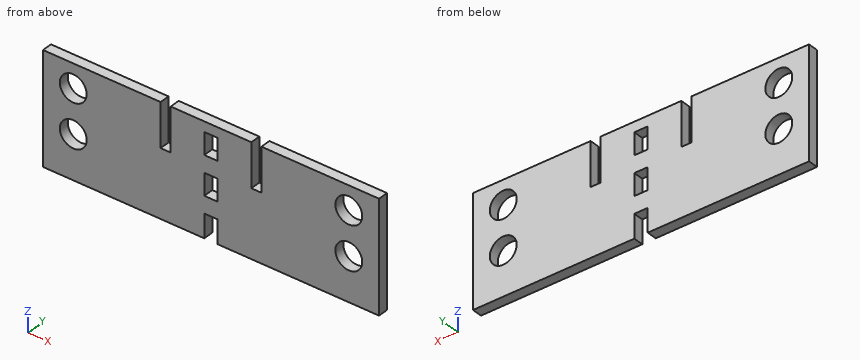
```python
from build123d import *

# Parameters (mm, degrees)
SKETCH_1_R          = 4
EXTRUDE_1_DEPTH     = 3
SKETCH_2_W          = 4
SKETCH_2_H          = 3
CUT_EXTRUDE_1_DEPTH = 3.33
SKETCH_3_W          = 24
SKETCH_3_H          = 13
EXTRUDE_2_DEPTH     = 3
SKETCH_4_W          = 35
SKETCH_4_H          = 13
EXTRUDE_3_DEPTH     = 3
SKETCH_5_R          = 4
CUT_EXTRUDE_2_DEPTH = 25
SKETCH_6_W          = 4
SKETCH_6_H          = 6.5
CUT_EXTRUDE_3_DEPTH = 25


with BuildPart() as part:
    # Эскиз1 → Бобышка-Вытянуть1 (new body)
    with BuildSketch(Plane(origin=(0, 0, 0), x_dir=(1, 0, 0), z_dir=(0, 1, 0))):
        Polygon((2, 10), (50, 10), (50, -10), (-50, -10), (-50, 10), (-2, 10), (-2, 6.32739691), (2, 6.32739691), align=None)
        with Locations(Location((-41, -3, 0), (0, 0, 270))):
            Circle(SKETCH_1_R, mode=Mode.SUBTRACT)
        with Locations(Location((41, -3, 0), (0, 0, 90))):
            Circle(SKETCH_1_R, mode=Mode.SUBTRACT)
    extrude(amount=EXTRUDE_1_DEPTH)

    # Эскиз2 → Вырез-Вытянуть1 (cut)
    with BuildSketch(Plane(origin=(0, 0, -6.32739691), x_dir=(-1, 0, 0), z_dir=(0, 0, -1))):
        with Locations((0, 1.5)):
            Rectangle(SKETCH_2_W, SKETCH_2_H)
    extrude(amount=-CUT_EXTRUDE_1_DEPTH, mode=Mode.SUBTRACT)

    # Эскиз3 → Бобышка-Вытянуть2 (add)
    with BuildSketch(Plane(origin=(0, 3, 0), x_dir=(1, 0, 0), z_dir=(0, 1, 0))):
        with Locations((0, -16.5)):
            Rectangle(SKETCH_3_W, SKETCH_3_H)
    extrude(amount=-EXTRUDE_2_DEPTH)

    # Эскиз4 → Бобышка-Вытянуть3 (add)
    with BuildSketch(Plane(origin=(0, 3, 0), x_dir=(1, 0, 0), z_dir=(0, 1, 0))):
        with Locations((-32.5, -16.5)):
            Rectangle(SKETCH_4_W, SKETCH_4_H)
        with Locations((32.5, -16.5)):
            Rectangle(SKETCH_4_W, SKETCH_4_H)
    extrude(amount=-EXTRUDE_3_DEPTH)

    # Эскиз5 → Вырез-Вытянуть2 (cut)
    with BuildSketch(Plane(origin=(0, 3, 0), x_dir=(1, 0, 0), z_dir=(0, 1, 0))):
        with Locations(Location((-41, -15.92753052, 0), (0, 0, 270))):
            Circle(SKETCH_5_R)
        with Locations(Location((41, -15.92753052, 0), (0, 0, 270))):
            Circle(SKETCH_5_R)
    extrude(amount=-CUT_EXTRUDE_2_DEPTH, mode=Mode.SUBTRACT)

    # Эскиз6 → Вырез-Вытянуть3 (cut)
    with BuildSketch(Plane(origin=(0, 3, 0), x_dir=(1, 0, 0), z_dir=(0, 1, 0))):
        with Locations((0, -5.25260309)):
            Rectangle(SKETCH_6_W, SKETCH_6_H)
        with Locations((0, -16.75260309)):
            Rectangle(SKETCH_6_W, SKETCH_6_H)
    extrude(amount=-CUT_EXTRUDE_3_DEPTH, mode=Mode.SUBTRACT)


solid = part.part
```
Check sheet for the modelled part. Datum: model origin and axes. Units: mm. Round coordinates to 2 decimals unless told otherwise and drop trailing zeros. Loops run counter-clockwise (first coordinate to the right, second up) from the corner with the lowest first, then second, coordinate; pieces in that order, holes last. Notation, with made-up numbers: M 87,5 L 121,5 A28 ccw 121,27 Z; hole C 39.5,31 d8. An arc over 180 degrees is marked long. Answer as a JSON object with one key per item and string values.
1. Section check D-D (z = 3). Record the boundary of the cut face in (x, y), plus the area to 3 significant figures.
Reply:
{"outline": "M -50,0 L -45,0 L -45,3 L -50,3 Z; M -37,0 L -2,0 L -2,3 L -37,3 Z; M 2,0 L 37,0 L 37,3 L 2,3 Z; M 45,0 L 50,0 L 50,3 L 45,3 Z", "area": "240 mm²"}
2. Section check B-B (x = -41). Record the boundary of the cut face in (y, z).
Reply:
{"outline": "M 0,-10 L 3,-10 L 3,-1 L 0,-1 Z; M 0,7 L 3,7 L 3,11.93 L 0,11.93 Z; M 0,19.93 L 3,19.93 L 3,23 L 0,23 Z"}
3. Scan lines: line 1 (X direction, y = 1.25, z = 3); line 2 (X direction, y = 1.9, z = 21.5); line 3 (X direction, y = 1.65, z = 0.5). Record each from-to range of solid material in increasing order.
Reply:
{"line 1": "x = -50 to -45, -37 to -2, 2 to 37, 45 to 50", "line 2": "x = -50 to -15, -12 to 12, 15 to 50", "line 3": "x = -50 to -44.12, -37.88 to 37.88, 44.12 to 50"}
4. Section check C-C (y = 1.5). Record the boundary of the cut face in (x, z).
Reply:
{"outline": "M -50,-10 L -2,-10 L -2,-3 L 2,-3 L 2,-10 L 50,-10 L 50,23 L 15,23 L 15,10 L 12,10 L 12,23 L -12,23 L -12,10 L -15,10 L -15,23 L -50,23 Z; hole C -41,3 d8; hole C -41,15.93 d8; hole M -2,2 L 2,2 L 2,8.5 L -2,8.5 Z; hole M -2,13.5 L 2,13.5 L 2,20 L -2,20 Z; hole C 41,3 d8; hole C 41,15.93 d8"}
5. Gauge pin test, flat ends, axial feed: P1, Ø0.9, axis at x = -13, y = 2, coming from the +Z side; P2, Ø0.9, axis at x = -1, y = 2, coming from the -Z side. Record the tip position at first contact, or that the pin passes through.
Reply:
{"P1": "stops at z = 10", "P2": "stops at z = -3"}
6. Section check A-A (z = -6.5). Record the boundary of the cut face in (x, y), plus the area to 3 significant figures.
Reply:
{"outline": "M -50,0 L -2,0 L -2,3 L -50,3 Z; M 2,0 L 50,0 L 50,3 L 2,3 Z", "area": "288 mm²"}
